CAD build for the part. Positions are in the model's coordinates, mm. Face numbers are marked on the shaded views. A direction names the side the tool comes from. Give positions to 0.01 mm unless a question says otherwise; leave off trailing zeros. Write each loop counter-clockwise with the first axis right and the second up, starting at its lowest first coordinate (ties: lowest second). Pieces come first, ordered by that corner, then holes. Notation, with made-up numbers: M -22,22 L 11,22 A29 ccw 11,55 Z; hole C 17.25,-32.5 d3. An arc over 180 degrees is marked long. One line per question, with ' | ' between items. Start each with the question number.
1. Cut at A-A, the plane y = -24. Write the cut outline in (x, z) (3 decimals), then the cut area to 3 significant figures.
2. Cut at D-D, the plane z = -16. Write the cut outline in (x, y).
3. Wall check: L1, parallel to Y at x = 72, z = -54; L2, parallel to X at y = -42.5, z = -29; L3, parallel to Z at x = -0.5, y = -17 (3 decimals). Give the ranges that are in metal, low to high.
4. Flat gauge pins, fed straight in: pin 1 (4.5 mm diameter, centred on y = -28, z = -75, fed in from +X); pin 2 (12 mm diameter, centred on x = -53, z = -57, fed in from -Y); pin 3 (8 mm diameter, centred on y = -44, z = -21.5, fed in from +X). Where does each tip first touch, or does it go through?
5. Cut at C-C, the plane z = -7.5. Write the cut outline in (x, y), then the cut area to 3 significant figures.
6. Pull direction Y, two halves, no side cores. Call the marked faces 4, 5 and 6: released by +Y, released by -Y, zero draft, split by the parting line, or undercut.
7. Cut at B-B, the plane x = -56. Write the cut outline in (y, z) (1 decimal), then the cut area to 3 significant figures.
8. Which spindle directions (+Z, -Z, +X, -X, +Y, -Y) get a long thin tool onto all of the face, cutting with end or side? Do the marked faces 1, 2 and 3. Say none if no direction does.
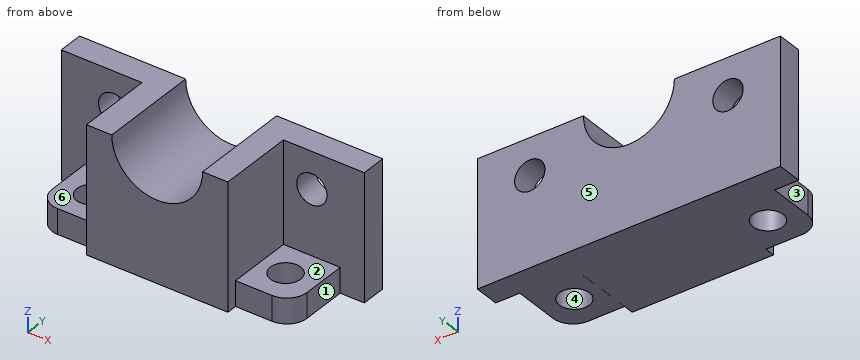
```python
from build123d import *

# Parameters (mm, degrees)
F1_DEPTH = 15.748
F4_DEPTH = 47.752
F6_R     = 9.525
F7_DEPTH = 15.748
F8_R     = 9.525
F9_DEPTH = 25.4


with BuildPart() as f1:
    # F0 (on Front) → F1 (new body)
    with BuildSketch(Plane.XZ):
        with BuildLine():
            ThreePointArc((28.575, 0), (0, -28.575), (-28.575, 0))
            Line((-28.575, 0), (-95.25, 0))
            Line((-95.25, 0), (-95.25, -79.375))
            Line((-95.25, -79.375), (95.25, -79.375))
            Line((95.25, -79.375), (95.25, 0))
            Line((95.25, 0), (28.575, 0))
        make_face()
    extrude(amount=F1_DEPTH)

    # F2 (on face) → F4 (join)
    with BuildSketch(Plane.XZ.offset(15.748)):
        with BuildLine():
            Line((-28.575, 0), (-44.470076, 0))
            Line((-44.470076, 0), (-44.470076, -79.375))
            Line((-44.470076, -79.375), (44.429924, -79.375))
            Line((44.429924, -79.375), (44.429924, 0))
            Line((44.429924, 0), (28.575, 0))
            ThreePointArc((28.575, 0), (0, -28.575), (-28.575, 0))
        make_face()
    extrude(amount=F4_DEPTH)

    # F6 (on offset) → F7 (join)
    with BuildSketch(Plane.XY.offset(-79.375)):
        with BuildLine():
            Line((-44.470076, -15.748), (-80.10444, -15.748))
            Line((-80.10444, -15.748), (-80.10444, -44.251695))
            ThreePointArc((-80.10444, -44.251695), (-76.384697, -53.231951), (-67.40444, -56.951695))
            Line((-67.40444, -56.951695), (-44.470076, -56.951695))
            Line((-44.470076, -56.951695), (-44.470076, -15.748))
        make_face()
        with Locations((-60.833134, -36.349847)):
            Circle(F6_R, mode=Mode.SUBTRACT)
        with BuildLine():
            ThreePointArc((67.40444, -56.951695), (76.384697, -53.231951), (80.10444, -44.251695))
            Line((80.10444, -44.251695), (80.10444, -15.748))
            Line((80.10444, -15.748), (44.470076, -15.748))
            Line((44.470076, -15.748), (44.470076, -56.951695))
            Line((44.470076, -56.951695), (67.40444, -56.951695))
        make_face()
        with Locations((60.833134, -36.349847)):
            Circle(F6_R, mode=Mode.SUBTRACT)
    extrude(amount=F7_DEPTH)

    # F8 (on face) → F9 (cut)
    with BuildSketch(Plane.XZ.offset(15.748)):
        with Locations((62.287258, -23.100371)):
            Circle(F8_R)
        with Locations((-62.287258, -23.100371)):
            Circle(F8_R)
    extrude(amount=-F9_DEPTH, mode=Mode.SUBTRACT)


solid = f1.part
```
Here are the results:
1) outline: M -80.104,-79.375 L 44.43,-79.375 L 44.43,0 L 28.575,0 A28.575 cw -28.575,0 L -44.47,0 L -44.47,-63.627 L -80.104,-63.627 Z; M 44.47,-79.375 L 80.104,-79.375 L 80.104,-63.627 L 44.47,-63.627 Z | area: 6,900 mm^2
2) outline: M -95.25,-15.75 L -68.64,-15.75 L -68.64,0 L -95.25,0 Z; M -55.94,-15.75 L -44.47,-15.75 L -44.47,-63.5 L -23.68,-63.5 L -23.68,0 L -55.94,0 Z; M 23.68,-63.5 L 44.43,-63.5 L 44.43,-15.75 L 55.94,-15.75 L 55.94,0 L 23.68,0 Z; M 68.64,-15.75 L 95.25,-15.75 L 95.25,0 L 68.64,0 Z
3) L1: -15.75 to 0 | L2: -44.47 to 44.43 | L3: -79.375 to -28.571
4) pin 1: x = 80.1 | pin 2: y = -15.75 | pin 3: x = 44.43
5) outline: M -95.25,-15.75 L -44.47,-15.75 L -44.47,-63.5 L -27.57,-63.5 L -27.57,0 L -95.25,0 Z; M 27.57,-63.5 L 44.43,-63.5 L 44.43,-15.75 L 95.25,-15.75 L 95.25,0 L 27.57,0 Z | area: 3,740 mm^2
6) face 4: undercut | face 5: released by +Y | face 6: zero draft
7) outline: M -57,-79.4 L -44.6,-79.4 L -44.6,-63.6 L -57,-63.6 Z; M -28.1,-79.4 L 0,-79.4 L 0,-30.3 L -15.7,-30.3 L -15.7,-63.6 L -28.1,-63.6 Z; M -15.7,-15.9 L 0,-15.9 L 0,0 L -15.7,0 Z | area: 1,420 mm^2
8) face 1: +Z, -Z, +X, -Y | face 2: +Z, +X, -Y | face 3: +Z, -Z, -X, -Y
